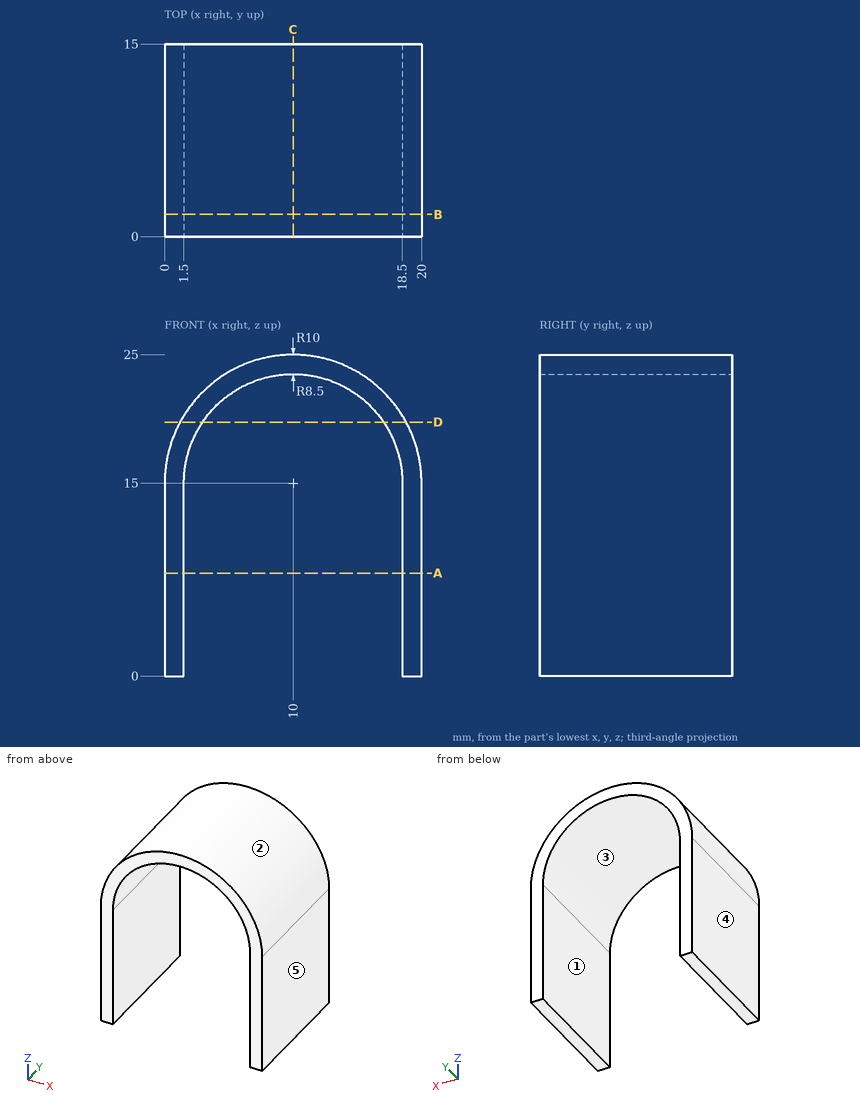
Answer from the drawing. Dimensions are ordinates in mm from the lowest x, y and z of the part. A direction names the side the tool comes from. Coordinates: 2 decimals unless noted, no trailing zeros. Write each loop counter-clockwise with the first axis right and the second up, starting at its lowest first coordinate (ties: lowest second). Pieces come first, ordered by that corner, then holes. Notation, with made-up numbers: M 82,54.25 L 88,54.25 A34 ccw 88,93.25 Z; hole C 10,40.5 d6. An arc over 180 degrees is marked long. Put each result on its own line as item: value. Start each with the question number.
1. A cutting plane is placed at A-A on z = 8. Write down the section's boundary in (x, y), then the cut area to 3 significant figures.
2. Consider line 1 (X direction, y = 7, z = 13); line 2 (X direction, y = 7.5, z = 22.75); line 3 (Z direction, x = 11.75, y = 8.75). Determine where each line is inside the solid, lowest interval first. Write a range as from..to.
3. Which of the six approach directions +Z, -Z, +X, -X, +Y, -Y give full straight-line access (tool end or side, diameter ignored) to the marked faces 1 and 2?
4. A cutting plane is placed at D-D on z = 19.75. Write down the section's boundary in (x, y).
5. For a pull along X with two mould halves and no side action, classify the marked faces 3, 4 and 5 as pulls with the +X half, pulls with the -X half, needs draft (parallel to the pull), parting line crosses it, or undercut.
6. Flat-ended cylindrical pins translate along their axes: P1, Ø1.5, axis at x = 5.5, y = 8.5, coming from the +Z side; P2, Ø2, axis at x = 16, y = 7, coming from the +Z side. Find the tip coordinate at first contact, or state that the pin passes through.
7. A cutting plane is placed at C-C on x = 10. Write down the section's boundary in (y, z), then the cut area to 3 significant figures.
8. A cutting plane is placed at B-B on y = 1.75. Write down the section's boundary in (x, z).
Resolved:
1. outline: M 0,0 L 1.5,0 L 1.5,15 L 0,15 Z; M 18.5,0 L 20,0 L 20,15 L 18.5,15 Z
1. area: 45.0 mm2
2. line 1: x = 0..1.5, 18.5..20
2. line 2: x = 3.68..6.51, 13.49..16.32
2. line 3: z = 23.32..24.85
3. face 1: -Z, +Y, -Y
3. face 2: +Z, +Y, -Y
4. outline: M 1.2,0 L 2.95,0 L 2.95,15 L 1.2,15 Z; M 17.05,0 L 18.8,0 L 18.8,15 L 17.05,15 Z
5. face 3: undercut
5. face 4: pulls with the -X half
5. face 5: pulls with the +X half
6. P1: stops at z = 24.27
6. P2: stops at z = 23.66
7. outline: M 0,23.5 L 15,23.5 L 15,25 L 0,25 Z
7. area: 22.5 mm2
8. outline: M 0,0 L 1.5,0 L 1.5,15 A8.5 cw 18.5,15 L 18.5,0 L 20,0 L 20,15 A10 ccw 0,15 Z
